Job drawing, mm, ordinate dimensions from the low corner. One solid piece. A direction names the side the tool comes from. Coordinates: 2 decimals unless noted, no trailing zeros. Write each loop counter-clockwise with the first axis right and the second up, starting at its lowest first coordinate (ties: lowest second). Pieces come first, ordered by that corner, then holes. Notation, with made-up numbers: (69, 51) - (127, 51) arc R10 cw to (127, 55) - close; hole circle Ø5 at (64.5, -39). An arc over 180 degrees is marked (long way). Put each result on its own line as item: value. Start each with the question number.
1. Drop flat-ended pins along their axis: P1, Ø7.5, axis at y = 6.35, z = 17.5, coming from the +X side; P2, Ø5.5, axis at x = 17.5, y = 6.35, coming from the +Z side; P3, Ø7.5, axis at x = 17.5, y = 6.35, coming from the +Z side; P4, Ø12, axis at x = 5, z = 5, coming from the -Y side. Give the stop position or say it passes through.
2. Saw through at C-C, the plane x = 22.5. Write the cut outline in (y, z) (3 decimals), plus the area to 3 significant figures.
3. Which spindle directions (+Z, -Z, +X, -X, +Y, -Y) get a long thin tool onto all of the face, cutting with end or side? Do the marked faces 4, 5 and 6. Say none if no direction does.
4. Drill centre lines: L1, parallel to Y at x = 17.5, z = 7.5; L2, parallel to X at y = 1.6, z = 17.5; L3, parallel to Y at x = 17.5, z = 19 (3 decimals). Where is each one in solid material? Low to high. Write a range as from..to.
5. Saw through at D-D, the plane y = 18.7. Write the cut outline in (x, z), plus the area to 3 significant figures.
6. Saw through at A-A, the plane y = 6.35. Write the cut outline in (x, z) (3 decimals).
7. Pull direction Z, two halves, no side cores. Call the marked faces 1, 2 and 3: released by +Z, released by -Z, zero draft, split by the parting line, or undercut.
8. Saw through at B-B, the plane z = 22. Write the cut outline in (x, y) (3 decimals).
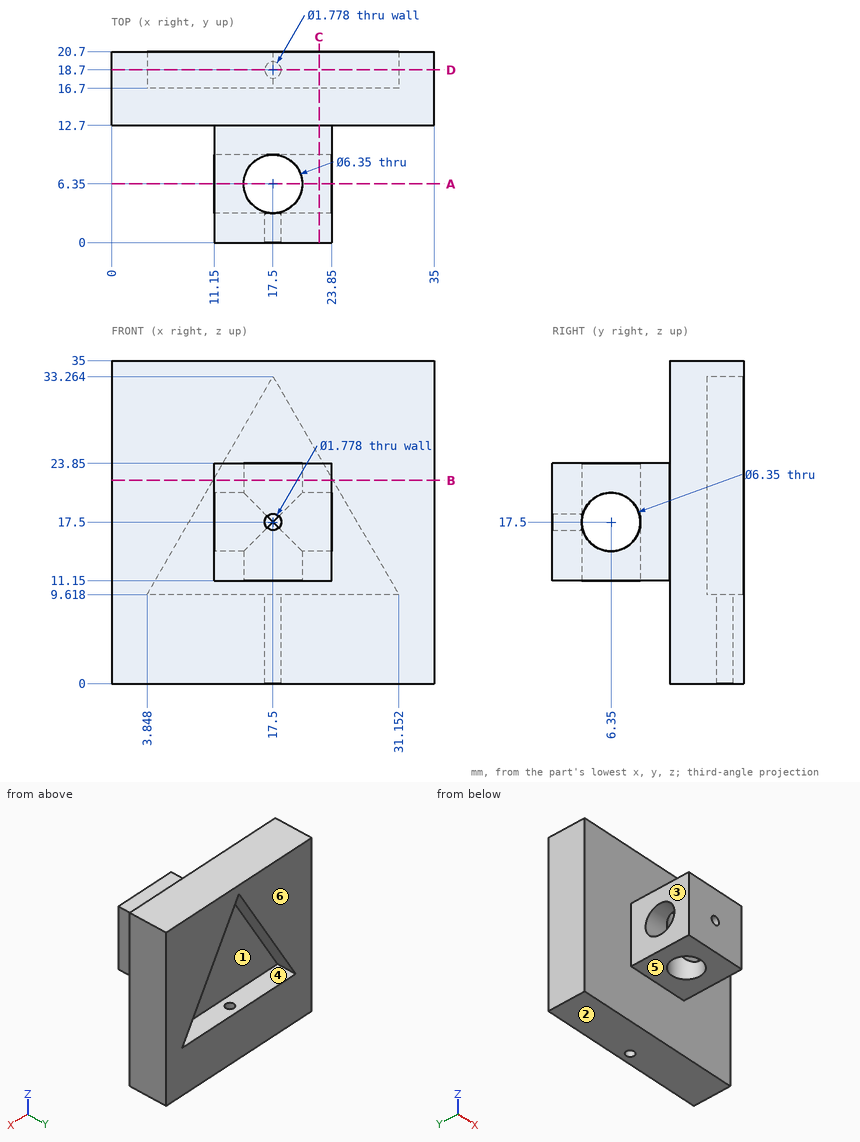
Final values:
1. P1: stops at x = 23.85
1. P2: passes through
1. P3: stops at z = 23.85
1. P4: stops at y = 12.7
2. outline: (0, 11.15) - (12.7, 11.15) - (12.7, 0) - (20.7, 0) - (20.7, 9.618) - (16.7, 9.618) - (16.7, 24.604) - (20.7, 24.604) - (20.7, 35) - (12.7, 35) - (12.7, 23.85) - (0, 23.85) - close; hole circle Ø6.35 at (6.35, 17.5)
2. area: 350 mm²
3. face 4: +Y
3. face 5: -Z, +X, -X, -Y
3. face 6: +Z, -Z, +X, -X, +Y
4. L1: y = 12.7..17.81, 19.59..20.7
4. L2: x = 11.15..16.61, 18.39..23.85
4. L3: y = 0..3.175, 9.525..16.7
5. outline: (0, 0) - (16.61, 0) - (16.61, 9.62) - (3.85, 9.62) - (17.5, 33.26) - (31.15, 9.62) - (18.39, 9.62) - (18.39, 0) - (35, 0) - (35, 35) - (0, 35) - close
5. area: 885 mm²
6. outline: (11.15, 11.15) - (14.325, 11.15) - (14.325, 14.325) - (11.15, 14.325) - close; (11.15, 20.675) - (14.325, 20.675) - (14.325, 23.85) - (11.15, 23.85) - close; (20.675, 11.15) - (23.85, 11.15) - (23.85, 14.325) - (20.675, 14.325) - close; (20.675, 20.675) - (23.85, 20.675) - (23.85, 23.85) - (20.675, 23.85) - close
7. face 1: undercut
7. face 2: released by -Z
7. face 3: zero draft
8. outline: (0, 12.7) - (11.15, 12.7) - (11.15, 0) - (23.85, 0) - (23.85, 12.7) - (35, 12.7) - (35, 20.7) - (24.003, 20.7) - (24.003, 16.7) - (10.997, 16.7) - (10.997, 20.7) - (0, 20.7) - close; hole circle Ø6.35 at (17.5, 6.35)
